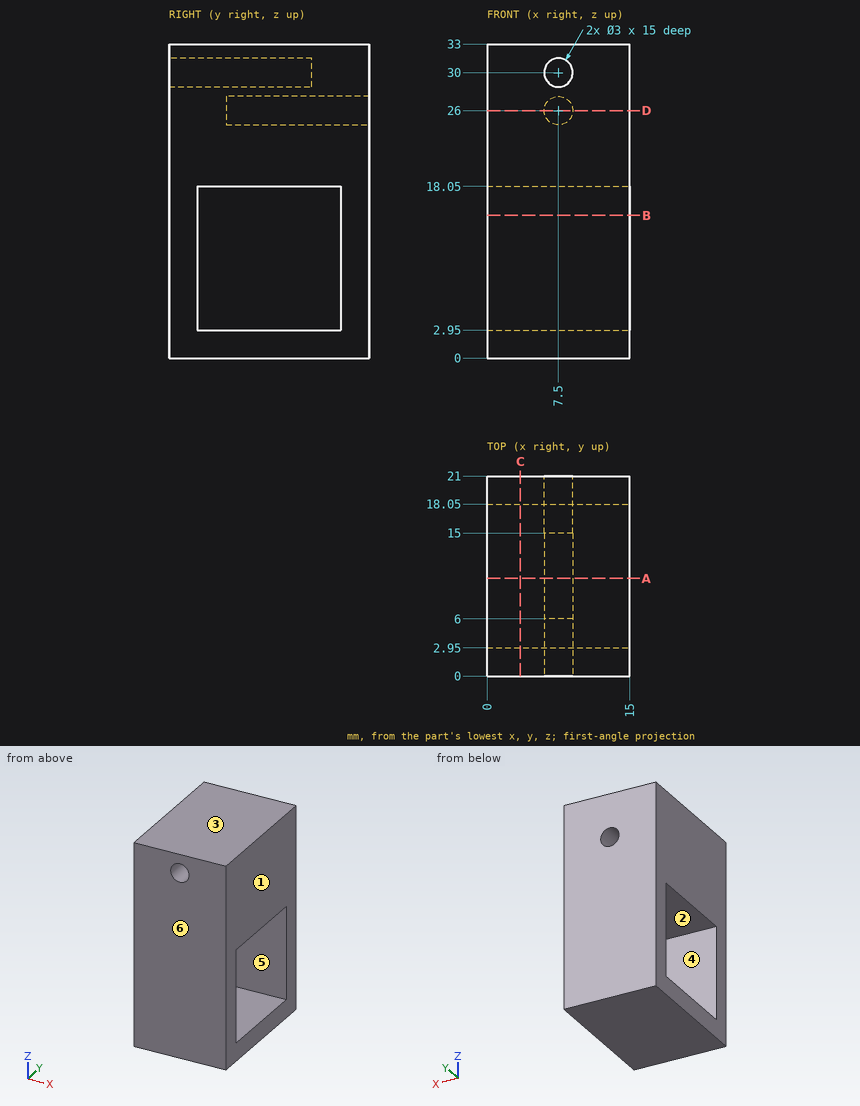
Study the drawing (mm; zero at the part's minimum x, y, z) and answer. A direction names the side the tool comes from. Give positions to 0.01 mm unless a question says otherwise; leave off trailing zeros. Loops run counter-clockwise (first coordinate to the right, second up) from the corner with the lowest first, then second, coordinate; pieces in that order, holes last. Notation, with made-up numbers: (48.5, 11.25) -> (92.5, 11.25) arc R37 cw to (92.5, 47.25) -> close; hole circle Ø6 at (75.5, 24). An arc over 180 degrees is marked (long way). Write item = value, one per line. Start each with the question number.
(1) Find the intervals of material crossed by probe 1 along Z at (x, y) = (9.25, 3); probe 2 along Y at (x, z) = (12.5, 17.5); probe 3 along X at (y, z) = (17, 26), in increasing order. Write a range as from..to.
(2) Find section A-A on y = 10.25. Give the vertices of the cut face in (x, z).
(3) Which of the six approach directions +Z, -Z, +X, -X, +Y, -Y give full straight-line access (tool end or side, diameter ignored) to the marked faces 1 and 2?
(4) The mould has two halves that part along Y. Classify the marked faces 3, 4, 5 and 6: +Y half, -Y half, draft (parallel to the pull), parting line (faces both ways), or undercut.
(5) Find section B-B on z = 15. Give the vertices of the cut face in (x, y).
(6) Find section C-C on x = 3.5. Give the vertices of the cut face in (y, z).
(7) Find section D-D on z = 26. Give the vertices of the cut face in (x, y).
From the geometry:
q1.probe_1 = 0..2.95, 18.05..33
q1.probe_2 = 0..2.95, 18.05..21
q1.probe_3 = 0..6, 9..15
q2.outline = (0, 0) -> (15, 0) -> (15, 2.95) -> (0, 2.95) -> close; (0, 18.05) -> (15, 18.05) -> (15, 33) -> (0, 33) -> close; hole circle Ø3 at (7.5, 26); hole circle Ø3 at (7.5, 30)
q3.face_1 = +Z, -Z, +X, +Y, -Y
q3.face_2 = +X, -X
q4.face_3 = draft
q4.face_4 = undercut
q4.face_5 = undercut
q4.face_6 = -Y half
q5.outline = (0, 0) -> (15, 0) -> (15, 2.95) -> (0, 2.95) -> close; (0, 18.05) -> (15, 18.05) -> (15, 21) -> (0, 21) -> close
q6.outline = (0, 0) -> (21, 0) -> (21, 33) -> (0, 33) -> close; hole (2.95, 2.95) -> (18.05, 2.95) -> (18.05, 18.05) -> (2.95, 18.05) -> close
q7.outline = (0, 0) -> (15, 0) -> (15, 21) -> (9, 21) -> (9, 6) -> (6, 6) -> (6, 21) -> (0, 21) -> close
